Model file for the job. Use its own axes, mm. Face numbers are marked on the shaded views. Coordinates: 2 decimals unless noted, no trailing zeros. Order: outer loops, then holes, each group sorted by start corner. A loop starts at its lowest first (then second) coordinate and runs counter-clockwise, first axis right, second up. Notation, with made-up numbers: M 68.5,78.25 L 121.5,78.25 A8 cw 121.5,90.25 Z; hole C 20,-1 d7. An arc over 180 degrees is marked long. Return JSON: item names as keys, results as strings.
```python
from build123d import *

# Parameters (mm, degrees)
SKETCH_R      = 1.64
SKETCH_R_2    = 1.9
PAD_DEPTH     = 2
SKETCH001_R   = 2.5
SKETCH001_R_2 = 1.64
PAD001_DEPTH  = 0.5


with BuildPart() as part:
    # Sketch → Pad (new body)
    with BuildSketch(Plane.XY):
        with BuildLine():
            ThreePointArc((3.784615, 1.576923), (0, 4.1), (-3.784615, 1.576923))
            Line((-3.784615, 1.576923), (-8.784615, -10.423077))
            ThreePointArc((-8.784615, -10.423077), (-8.41141, -14.274265), (-5.000015, -16.1))
            Line((-5.000015, -16.1), (5, -16.1))
            ThreePointArc((5, -16.1), (8.411406, -14.274271), (8.784615, -10.423077))
            Line((8.784615, -10.423077), (3.784615, 1.576923))
        make_face()
        with Locations((-5, -12)):
            Circle(SKETCH_R, mode=Mode.SUBTRACT)
        with Locations((5, -12)):
            Circle(SKETCH_R, mode=Mode.SUBTRACT)
        Circle(SKETCH_R_2, mode=Mode.SUBTRACT)
    extrude(amount=-PAD_DEPTH)

    # Sketch001 (on Face11 of Pad) → Pad001 (join)
    with BuildSketch(Plane(origin=(0, 0, -2), x_dir=(1, 0, 0), z_dir=(0, 0, -1))):
        with Locations((-5, 12)):
            Circle(SKETCH001_R)
        with Locations((-5, 12)):
            Circle(SKETCH001_R_2, mode=Mode.SUBTRACT)
        with Locations((5, 12)):
            Circle(SKETCH001_R)
        with Locations((5, 12)):
            Circle(SKETCH001_R_2, mode=Mode.SUBTRACT)
    extrude(amount=PAD001_DEPTH)


solid = part.part
```
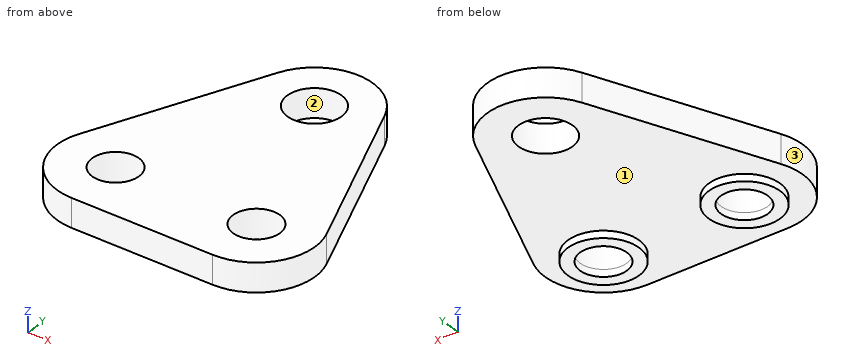
Item 1: Pull direction Y, two halves, no side cores. Call the marked faces 1, 2 and 3: +Y half, -Y half, draft (parallel to the pull), parting line (faces both ways), or undercut.
Check result:
{"face 1": "draft", "face 2": "undercut", "face 3": "parting line"}
Item 2: Wall check: line 1 (X direction, y = -12, z = -2.4); line 2 (Y direction, x = 0, z = -1.05); line 3 (X direction, y = -13.25, z = -1.2). Give the ranges that are in metal, low to high.
Check result:
{"line 1": "x = -7.5 to -6.64, -3.36 to -2.5, 2.5 to 3.36, 6.64 to 7.5", "line 2": "y = -16.1 to -1.9, 1.9 to 4.1", "line 3": "x = -8.9 to -6.06, -3.94 to 3.94, 6.06 to 8.9"}
Item 3: Saw through at C-C (z = -1.1). Write the cut outline in (x, y), and give its area (3 significant figures).
Check result:
{"outline": "M -8.78,-10.42 A4.1 ccw -5,-16.1 L 5,-16.1 A4.1 ccw 8.78,-10.42 L 3.78,1.58 A4.1 ccw -3.78,1.58 Z; hole C -5,-12 d3.28; hole C 0,0 d3.8; hole C 5,-12 d3.28", "area": "232 mm2"}
Item 4: Saw through at B-B (y = -12). Write the cut outline in (x, z), and give its area (3 significant figures).
Check result:
{"outline": "M -9.1,-2 L -7.5,-2 L -7.5,-2.5 L -6.64,-2.5 L -6.64,0 L -9.1,0 Z; M -3.36,-2.5 L -2.5,-2.5 L -2.5,-2 L 2.5,-2 L 2.5,-2.5 L 3.36,-2.5 L 3.36,0 L -3.36,0 Z; M 6.64,-2.5 L 7.5,-2.5 L 7.5,-2 L 9.1,-2 L 9.1,0 L 6.64,0 Z", "area": "25.0 mm2"}
Item 5: Saw through at D-D (y = -0.5). Write the cut outline in (x, z).
Check result:
{"outline": "M -4.65,-2 L -1.83,-2 L -1.83,0 L -4.65,0 Z; M 1.83,-2 L 4.65,-2 L 4.65,0 L 1.83,0 Z"}
Item 6: Saw through at A-A (x = 0). Write the cut outline in (y, z), and give its area (3 significant figures).
Check result:
{"outline": "M -16.1,-2 L -1.9,-2 L -1.9,0 L -16.1,0 Z; M 1.9,-2 L 4.1,-2 L 4.1,0 L 1.9,0 Z", "area": "32.8 mm2"}
